The listing builds one solid part. Answer for the finished solid, in the listing's coordinates (mm). Round coordinates to 2 decimals unless told otherwise and drop trailing zeros. Loops run counter-clockwise (first coordinate to the right, second up) from the corner with the lowest first, then second, coordinate; pieces in that order, holes last. Notation, with made-up numbers: (77.25, 23) -> (126.25, 23) arc R27 ccw to (126.25, 56) -> close; hole circle Ø11 at (46, 22). An arc over 180 degrees is marked (long way). One line per question, with ' | ' between items.
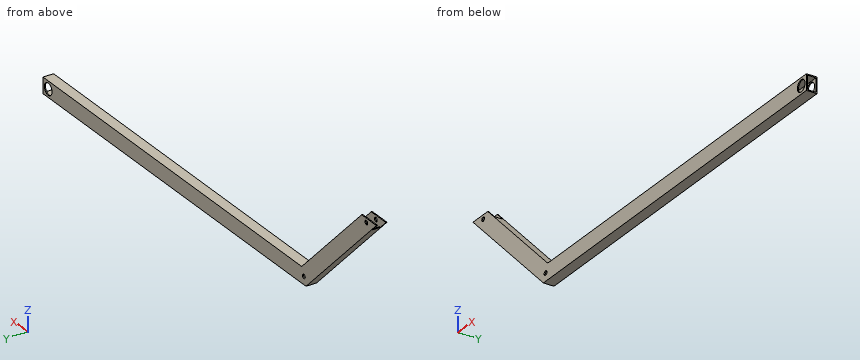
Solid Edge part; units mm, degrees
sketch "Sketch1" plane through (0, 0, 0) normal (0, -1, 0) x (1, 0, 0)
  line L0 (-166.1701, 187.3833) -> (6.2132, 15)
  line L1 (6.2132, 15) -> (750, 15)
  line L2 (750, -15) -> (750, 15)
  line L3 (750, -15) -> (-6.2132, -15)
  line L4 (-208.5965, 187.3833) -> (-6.2132, -15)
  line L5 (-166.1701, 187.3833) -> (-208.5965, 187.3833)
extrude "Protrusion1" add sketch "Sketch1" against normal blind 20
shell "Thinwall_1" thickness 2 removed faces 2 at (750, 16.4667, -10.3) at (-172.8169, 16.4667, 187.3833)
sketch "Sketch2" plane through (0, 0, 0) normal (0, -1, 0) x (1, 0, 0)
  circle A0 centre (-179.491, 179.491) radius 4
extrude "ExtrudedCutout_1" cut sketch "Sketch2" against normal blind 71.5444
sketch "Sketch3" plane through (0, 0, 0) normal (0, -1, 0) x (1, 0, 0)
  circle A0 centre (0, 0) radius 4
extrude "ExtrudedCutout_2" cut sketch "Sketch3" against normal blind 129.6912
sketch "Sketch4" plane through (0, 0, 0) normal (0, -1, 0) x (1, 0, 0)
  circle A0 centre (735, 0) radius 11
extrude "ExtrudedCutout_3" cut sketch "Sketch4" against normal blind 104.4525
sketch "Sketch5" plane through (0, 0, 0) normal (1, 0, 0) x (0, 1, 0)
  line L0 (18, 171.3833) -> (18, 187.3833)
  line L1 (2, 187.3833) -> (18, 187.3833)
  line L2 (2, 187.3833) -> (2, 171.3833)
  line L3 (2, 171.3833) -> (18, 171.3833)
extrude "ExtrudedCutout_4" cut sketch "Sketch5" against normal blind 277.745
Q1. A cutting plane is placed at D-D on z = 45. Give the vertices of the cut face in (x, y), plus the area to 3 significant figures.
Numbers:
outline: (-66.21, 0) -> (-23.79, 0) -> (-23.79, 20) -> (-66.21, 20) -> close; hole (-63.38, 2) -> (-26.62, 2) -> (-26.62, 18) -> (-63.38, 18) -> close | area: 260 mm^2
Q2. A cutting plane is placed at A-A on x = 735. Give the vertices of the cut face in (y, z), plus the area to 3 significant figures.
Numbers:
outline: (0, -15) -> (20, -15) -> (20, -11) -> (18, -11) -> (18, -13) -> (2, -13) -> (2, -11) -> (0, -11) -> close; (0, 11) -> (2, 11) -> (2, 13) -> (18, 13) -> (18, 11) -> (20, 11) -> (20, 15) -> (0, 15) -> close | area: 96.0 mm^2
Q3. A cutting plane is placed at B-B on y = 9.5. Give the vertices of the cut face in (x, z).
Numbers:
outline: (-192.6, 171.38) -> (-6.21, -15) -> (750, -15) -> (750, -13) -> (-5.38, -13) -> (-189.77, 171.38) -> close; (-153, 171.38) -> (5.38, 13) -> (750, 13) -> (750, 15) -> (6.21, 15) -> (-150.17, 171.38) -> close
Q4. Find the intervals of material crossed by line 1 (Z direction, x = 108.5, y = 4.25); line 2 (Z direction, x = 735, y = 0.5); line 3 (Y direction, x = 192, z = -5), in increasing order. Write a range as from..to.
Numbers:
line 1: -15..-13, 13..15 | line 2: -15..-11, 11..15 | line 3: 0..2, 18..20
Q5. Given pin 1 Ø8 at (y, z) = (16, 17) entering from -X; pin 2 Ø1 at (y, z) = (16.5, 128) entering from +X; pin 3 Ø5 at (x, y) = (195.5, 13) entering from +Z; pin 4 Ø6.5 at (x, z) = (0, 0) entering from +Y, each flat-ended and moving along its own axis, determine where each tip first touches the part or whether it passes through.
Numbers:
pin 1: x = -42.21 | pin 2: x = -106.29 | pin 3: z = 15 | pin 4: through
Q6. A cutting plane is placed at C-C on x = 614.5. Give the vertices of the cut face in (y, z).
Numbers:
outline: (0, -15) -> (20, -15) -> (20, 15) -> (0, 15) -> close; hole (2, -13) -> (18, -13) -> (18, 13) -> (2, 13) -> close
